Geometry: final body of the model. Coordinates: model frame, mm. Give positions to 0.01 mm unless a question says otherwise; leave off trailing zeros. Write each loop counter-clockwise with the first axis right and the second up, starting at its lowest first coordinate (ties: lowest second). Pieces come first, ordered by that corner, then holes.
from build123d import *

# Parameters (mm, degrees)
SKETCH1_W                       = 50
SKETCH1_H                       = 50
BOSS_EXTRUDE1_DEPTH             = 60
F_8_0MM_DOWEL_HOLE1_D           = 8
F_8_0MM_DOWEL_HOLE1_CSINK_D     = 8.05
F_8_0MM_DOWEL_HOLE1_CSINK_ANGLE = 90


with BuildPart() as part:
    # Sketch1 → Boss-Extrude1 (new body)
    with BuildSketch(Plane(origin=(0, 0, 0), x_dir=(1, 0, 0), z_dir=(0, 1, 0))):
        Rectangle(SKETCH1_W, SKETCH1_H)
    extrude(amount=BOSS_EXTRUDE1_DEPTH)

    # Ø8.0mm Dowel Hole1 (through all)
    with Locations(Plane(origin=(25, 0, 0), x_dir=(0, 0, -1), z_dir=(1, 0, 0))):
        with Locations((0, 52.184072135)):
            CounterSinkHole(F_8_0MM_DOWEL_HOLE1_D / 2, F_8_0MM_DOWEL_HOLE1_CSINK_D / 2, counter_sink_angle=F_8_0MM_DOWEL_HOLE1_CSINK_ANGLE)


solid = part.part
Q1. Section B-B on x = -20.5. Output: boundary loops of the cut face in (y, z).
Filled sheet:
outline: (0, -25) - (60, -25) - (60, 25) - (0, 25) - close; hole circle Ø8 at (52.18, 0)
Q2. Ray query, line 1 along Y through (x, z) = (-4.5, 0); line 2 along Z through (x, y) = (2, 55.5); line 3 along Z through (x, y) = (-3, 53). Return the intervals inside material, ascending.
Filled sheet:
line 1: y = 0 to 48.18, 56.18 to 60
line 2: z = -25 to -2.24, 2.24 to 25
line 3: z = -25 to -3.92, 3.92 to 25
Q3. Pull-direction query (Y, two-part tool) for faces 1 (the cylindrical face through (-0.36, 56.15, -0.52)), 2 (the flat face through (0, 0, 0)), 3 (the flat face through (-25, 30, 0)); classes: released by +Y, released by -Y, zero draft, split by the parting line, or undercut.
Filled sheet:
face 1: undercut
face 2: released by -Y
face 3: zero draft
Q4. Section A-A on z = 0. Output: boundary loops of the cut face in (x, y) (3 decimals), plus the area to 3 significant figures.
Filled sheet:
outline: (-25, 0) - (25, 0) - (25, 48.159) - (24.975, 48.184) - (-25, 48.184) - close; (-25, 56.184) - (24.975, 56.184) - (25, 56.209) - (25, 60) - (-25, 60) - close
area: 2,600 mm2
Q5. Pin query (flat end, axial travel): P1, Ø5, axis at y = 52.18, z = 0, coming from the -X side. Return the tip coordinate at first contact, or that it passes through.
Filled sheet:
P1: passes through
